```python
from build123d import *

# Parameters (mm, degrees)
SKETCH1_W           = 139
SKETCH1_H           = 83
SKETCH1_R           = 1.6
SKETCH1_R_2         = 3.1
SKETCH1_R_3         = 1.25
SKETCH1_R_4         = 3.75
SKETCH1_R_5         = 5.1
SKETCH1_W_2         = 2.7
SKETCH1_H_2         = 1.2
SKETCH1_W_3         = 1.2
SKETCH1_H_3         = 2.7
SKETCH1_W_4         = 2.2
SKETCH1_H_4         = 1.1
BOSS_EXTRUDE1_DEPTH = 3


with BuildPart() as part:
    # Sketch1 → Boss-Extrude1 (new body)
    with BuildSketch(Plane.XY):
        with Locations((69.5, 41.5)):
            Rectangle(SKETCH1_W, SKETCH1_H)
        with Locations((4, 55.5)):
            Circle(SKETCH1_R, mode=Mode.SUBTRACT)
        with Locations((135, 55.5)):
            Circle(SKETCH1_R, mode=Mode.SUBTRACT)
        with Locations((135, 11.5)):
            Circle(SKETCH1_R, mode=Mode.SUBTRACT)
        with Locations((4, 11.5)):
            Circle(SKETCH1_R, mode=Mode.SUBTRACT)
        with Locations((48.65436543, 14.544998484)):
            Circle(SKETCH1_R, mode=Mode.SUBTRACT)
        with Locations((24.475038928, 25.666634818)):
            Circle(SKETCH1_R_2, mode=Mode.SUBTRACT)
        with Locations((135, 77.5)):
            Circle(SKETCH1_R_3, mode=Mode.SUBTRACT)
        with Locations((4, 77.5)):
            Circle(SKETCH1_R_3, mode=Mode.SUBTRACT)
        with Locations((74.615565323, 25.361106272)):
            Circle(SKETCH1_R_2, mode=Mode.SUBTRACT)
        with Locations((106.932598637, 14.544998484)):
            Circle(SKETCH1_R_2, mode=Mode.SUBTRACT)
        with Locations((47.55436543, 35.562774654)):
            Circle(SKETCH1_R_4, mode=Mode.SUBTRACT)
        with Locations((69.5, 69.231811206)):
            Circle(SKETCH1_R_5, mode=Mode.SUBTRACT)
        with Locations((113.858121324, 61.952726152)):
            Circle(SKETCH1_R, mode=Mode.SUBTRACT)
        with Locations((90.80059856, 46.596907859)):
            Circle(SKETCH1_R_2, mode=Mode.SUBTRACT)
        with Locations((105.80059856, 46.596907859)):
            Circle(SKETCH1_R_2, mode=Mode.SUBTRACT)
        with Locations((120.80059856, 46.596907859)):
            Circle(SKETCH1_R_2, mode=Mode.SUBTRACT)
        with Locations((74.615565323, 19.361106272)):
            Rectangle(SKETCH1_W_2, SKETCH1_H_2, mode=Mode.SUBTRACT)
        with Locations((24.475038928, 19.666634818)):
            Rectangle(SKETCH1_W_2, SKETCH1_H_2, mode=Mode.SUBTRACT)
        with Locations((112.932598637, 14.544998484)):
            Rectangle(SKETCH1_W_3, SKETCH1_H_3, mode=Mode.SUBTRACT)
        with Locations((47.55436543, 29.312774654)):
            Rectangle(SKETCH1_W_4, SKETCH1_H_4, mode=Mode.SUBTRACT)
        with Locations((90.80059856, 40.596907859)):
            Rectangle(SKETCH1_W_2, SKETCH1_H_2, mode=Mode.SUBTRACT)
        with Locations((105.80059856, 40.596907859)):
            Rectangle(SKETCH1_W_2, SKETCH1_H_2, mode=Mode.SUBTRACT)
        with Locations((120.80059856, 40.596907859)):
            Rectangle(SKETCH1_W_2, SKETCH1_H_2, mode=Mode.SUBTRACT)
    extrude(amount=BOSS_EXTRUDE1_DEPTH)


solid = part.part
```
CAD build for the part. Positions are in the model's coordinates, mm. Give positions to 0.01 mm unless a question says otherwise; leave off trailing zeros. Write each loop counter-clockwise with the first axis right and the second up, starting at its lowest first coordinate (ties: lowest second). Pieces come first, ordered by that corner, then holes. Notation, with made-up numbers: M 16.25,-28.5 L 71.25,-28.5 A28 ccw 71.25,-8.5 Z; hole C 39,-21 d7. An arc over 180 degrees is marked long. Return JSON: item names as keys, results as strings. Group by question number.
(1) Mould opens along Y. For faces 1 (the face through (69, 0, 1)), 2 (the face through (106, 39.997, 1)), 3 (the face through (139, 41, 1)) say: pulls with the +Y half, pulls with the -Y half, needs draft (parallel to the pull), parting line crosses it, or undercut.
(2) Drill centre lines: L1, parallel to Y at x = 135, z = 1.25; L2, parallel to X at y = 77.5, z = 1.9; L3, parallel to X at y = 25, z = 2.1. Where is each one in solid material? Low to high. Write a range as [from, to].
(3) Band-saw the part on B-B (y = 55.5). Give the cut face in (x, z), and give its area (3 significant figures).
(4) Band-saw the part on D-D (y = 24). Give the cut face in (x, z), and give its area (3 significant figures).
(5) Flat gauge pins, fed straight in: pin 1 Ø6 at (x, y) = (90, 55.5) entering from -Z; pin 2 Ø5 at (x, y) = (24.48, 25.67) entering from +Z. Where does each tip first touch, or does it go through?
(6) Band-saw the part on C-C (y = 73). Give the cut face in (x, z).
(7) Band-saw the part on A-A (x = 69.5). Give the cut face in (y, z), and give its area (3 significant figures).
Entries:
{
 "1": {"face 1": "pulls with the -Y half", "face 2": "undercut", "face 3": "needs draft"},
 "2": {"L1": "y = [0, 9.9], [13.1, 53.9], [57.1, 76.25], [78.75, 83]", "L2": "x = [0, 2.75], [5.25, 133.75], [136.25, 139]", "L3": "x = [0, 21.45], [27.5, 71.54], [77.69, 139]"},
 "3": {"outline": "M 0,0 L 2.4,0 L 2.4,3 L 0,3 Z; M 5.6,0 L 133.4,0 L 133.4,3 L 5.6,3 Z; M 136.6,0 L 139,0 L 139,3 L 136.6,3 Z", "area": "398 mm^2"},
 "4": {"outline": "M 0,0 L 21.86,0 L 21.86,3 L 0,3 Z; M 27.09,0 L 71.83,0 L 71.83,3 L 27.09,3 Z; M 77.4,0 L 139,0 L 139,3 L 77.4,3 Z", "area": "385 mm^2"},
 "5": {"pin 1": "stops at z = 0", "pin 2": "passes through"},
 "6": {"outline": "M 0,0 L 66.06,0 L 66.06,3 L 0,3 Z; M 72.94,0 L 139,0 L 139,3 L 72.94,3 Z"},
 "7": {"outline": "M 0,0 L 64.13,0 L 64.13,3 L 0,3 Z; M 74.33,0 L 83,0 L 83,3 L 74.33,3 Z", "area": "218 mm^2"}
}
